Geometry check sheet. Reference: the model listing, model coordinates, mm. A direction names the side the tool comes from. Round coordinates to 2 decimals unless told otherwise and drop trailing zeros. Write each loop counter-clockwise with the first axis right and the second up, starting at its lowest first coordinate (ties: lowest second). Pieces come first, ordered by that corner, then holes. Notation, with made-up numbers: (29.25, 23) -> (39.25, 23) arc R18 ccw to (39.25, 34) -> close; hole circle Ø2 at (71.25, -27). An arc over 180 degrees is marked (long way). Put each result on its own line as item: value. Start each with the question number.
from build123d import *

# Parameters (mm, degrees)
ESQUISSE1_R             = 15
BASE_EXTRUSION_DEPTH    = 400
CHANFREIN1_SIZE         = 1
ENL_V_MAT_EXTRU_1_DEPTH = 10
ESQUISSE3_W             = 50
ESQUISSE3_H             = 10
ENL_V_MAT_EXTRU_2_DEPTH = 10


with BuildPart() as part:
    # Esquisse1 → Base-Extrusion (new body)
    with BuildSketch(Plane.XY):
        with Locations(Location((0, 0, 0), (0, 0, 184.920671017))):
            Circle(ESQUISSE1_R)
    extrude(amount=BASE_EXTRUSION_DEPTH)

    # Chanfrein1
    chanfrein1_edges = [part.edges().sort_by_distance(p)[0] for p in [
        (14.944716223, 1.286645645, 400),
    ]]
    chamfer(chanfrein1_edges, length=CHANFREIN1_SIZE)

    # Esquisse2 → Enlèv. mat.-Extru.1 (cut)
    with BuildSketch(Plane.XY.offset(400)):
        Polygon((17.08733053, 32.74178837), (-26.801262557, -13.882147509), (-38.674413155, -3.843373525), (5.782041814, 43.38381605), align=None)
    extrude(amount=-ENL_V_MAT_EXTRU_1_DEPTH, mode=Mode.SUBTRACT)

    # Esquisse3 → Enlèv. mat.-Extru.2 (cut)
    with BuildSketch(Plane(origin=(0, 0, 0), x_dir=(-1, 0, 0), z_dir=(0, 0, -1))):
        with Locations((5, 15)):
            Rectangle(ESQUISSE3_W, ESQUISSE3_H)
    extrude(amount=-ENL_V_MAT_EXTRU_2_DEPTH, mode=Mode.SUBTRACT)


solid = part.part
(1) Sectioned sample at A-A (z = 107.5). Record the cut outline in (x, y).
(2) Material ranges on L1, parallel to X at y = 5.5, z = 275; L2, parallel to Y at x = 1, z = 102.5; L3, parallel to Z at x = -10, y = 8, recorded low to high. Write a range as from..to.
(3) Set-up check for faces 1 (the flat face through (0, 0, 400)), 2 (the flat face through (0, 10, 5)), 3 (the flat face through (-7.17, 6.97, 395.07)): record each of +Z, -Z, +X, -X, +Y, -Y from which the full face is reachable in a straight line by a thin tool's end or side.
(4) Go/stop test with flat-tipped pins: pin 1 Ø8 at (x, z) = (3, 7) entering from +Y; pin 2 Ø8 at (y, z) = (7, 260) entering from -X; pin 3 Ø8 at (y, z) = (5.5, 336) entering from +X. Record where each tip stops, or that it passes through.
Found:
1. outline: circle Ø30 at (0, 0)
2. L1: -13.96..13.96
2. L2: -14.97..14.97
2. L3: 0..390
3. face 1: +Z, +X, -X, +Y, -Y
3. face 2: -Z, +X, -X, +Y
3. face 3: +Z, -X, +Y
4. pin 1: y = 15
4. pin 2: x = -14.7
4. pin 3: x = 14.92
